from build123d import *

# Parameters (mm, degrees)
BOSS_EXTRUDE1_DEPTH = 11
CHAMFER1_SIZE       = 3
SKETCH2_R           = 1.5
CUT_EXTRUDE1_DEPTH  = 39.050256569


with BuildPart() as part:
    # Sketch1 → Boss-Extrude1 (new body)
    with BuildSketch(Plane.XY):
        Polygon((-26.955, 0), (-17.955, 0), (-17.955, 24.5), (17.955, 24.5), (17.955, 0), (26.955, 0), (26.955, 3), (20.955, 3), (20.955, 27.5), (-20.955, 27.5), (-20.955, 3), (-26.955, 3), align=None)
    extrude(amount=BOSS_EXTRUDE1_DEPTH)

    # Chamfer1
    chamfer1_edges = [part.edges().sort_by_distance(p)[0] for p in [
        (-26.955, 1.5, 0),
        (26.955, 1.5, 0),
        (26.955, 1.5, 11),
        (-26.955, 1.5, 11),
    ]]
    chamfer(chamfer1_edges, length=CHAMFER1_SIZE)

    # Sketch2 → Cut-Extrude1 (cut, through all)
    with BuildSketch(Plane(origin=(0, 3, 0), x_dir=(1, 0, 0), z_dir=(0, 1, 0))):
        with Locations(Location((-23.955, -5.5, 0), (0, 0, 180))):
            Circle(SKETCH2_R)
        with Locations((23.955, -5.5)):
            Circle(SKETCH2_R)
    extrude(amount=-CUT_EXTRUDE1_DEPTH, mode=Mode.SUBTRACT)


solid = part.part
Work out the finished part from the listing and answer in its coordinate system (mm). A direction names the side the tool comes from. Round coordinates to 2 decimals unless told otherwise and drop trailing zeros. Loops run counter-clockwise (first coordinate to the right, second up) from the corner with the lowest first, then second, coordinate; pieces in that order, holes last. Notation, with made-up numbers: (-0.5, 24.5) - (41.5, 24.5) arc R22 cw to (41.5, 33.5) - close; hole circle Ø4 at (37, 74). An arc over 180 degrees is marked (long way). One line per item, written item: value.
Q1. Find section B-B on y = 7.5. Give the vertices of the cut face in (x, z) (3 decimals), and give its area (3 significant figures).
Check values:
outline: (-20.955, 0) - (-17.955, 0) - (-17.955, 11) - (-20.955, 11) - close; (17.955, 0) - (20.955, 0) - (20.955, 11) - (17.955, 11) - close
area: 66.0 mm2
Q2. Each of these flat-tipped pins is pushed along its axis until it touches: pin 1 Ø3 at (x, z) = (23, 4.5) entering from +Y; pin 2 Ø3.5 at (y, z) = (16, 4) entering from -X (3 decimals); pin 3 Ø4 at (x, z) = (8.5, 9.5) entering from -Y; pin 4 Ø2.5 at (x, z) = (-23.955, 5.5) entering from -Y. Where does it stop, or does it pass through?
Check values:
pin 1: y = 3
pin 2: x = -20.955
pin 3: y = 24.5
pin 4: through
Q3. The mould has two halves that part along X. Classify faces 1 (the flat face through (-23, 3, 7)), 2 (the flat face through (0, 24.5, 5)), 3 (the flat face through (25.434, 1.479, 1.479)): +X half, -X half, draft (parallel to the pull), parting line (faces both ways), or undercut.
Check values:
face 1: draft
face 2: undercut
face 3: +X half
Q4. For faces 4 (the flat face through (23, 3, 4)), 5 (the flat face through (-20.955, 15, 5)), 6 (the flat face through (-17.955, 12, 5)), determine the directions among +Z, -Z, +X, -X, +Y, -Y from which every point of the face is accessible in a straight line to the end or side of a thin tool.
Check values:
face 4: +Z, -Z, +X, +Y
face 5: +Z, -Z, -X, +Y
face 6: +Z, -Z, -Y
Q5. Find section A-A on z = 5.5. Give the vertices of the cut face in (x, y) (3 decimals).
Check values:
outline: (-26.955, 0) - (-25.455, 0) - (-25.455, 3) - (-26.955, 3) - close; (-22.455, 0) - (-17.955, 0) - (-17.955, 24.5) - (17.955, 24.5) - (17.955, 0) - (22.455, 0) - (22.455, 3) - (20.955, 3) - (20.955, 27.5) - (-20.955, 27.5) - (-20.955, 3) - (-22.455, 3) - close; (25.455, 0) - (26.955, 0) - (26.955, 3) - (25.455, 3) - close
Q6. Straight lines are drawn through the part: probe 1 along X at (y, z) = (9.25, 5.75) (3 decimals); probe 2 along Y at (x, z) = (9, 3.25); probe 3 along X at (y, z) = (1.75, 10.25) (3 decimals). For each, find the intervals that lie inside material, in ascending order.
Check values:
probe 1: -20.955 to -17.955, 17.955 to 20.955
probe 2: 24.5 to 27.5
probe 3: -24.705 to -17.955, 17.955 to 24.705
Q7. Find section C-C on x = 23. Give the vertices of the cut face in (y, z).
Check values:
outline: (0, 0) - (3, 0) - (3, 4.34) - (0, 4.34) - close; (0, 6.66) - (3, 6.66) - (3, 11) - (0, 11) - close
Q8. Find section D-D on x = -4.5. Give the vertices of the cut face in (y, z), and give its area (3 significant figures).
Check values:
outline: (24.5, 0) - (27.5, 0) - (27.5, 11) - (24.5, 11) - close
area: 33.0 mm2
